from build123d import *

# Parameters (mm, degrees)
SKETCH1_W                                     = 120
SKETCH1_H                                     = 36.5
BOSS_EXTRUDE1_DEPTH                           = 3
CUT_EXTRUDE1_DEPTH                            = 4
CSK_FOR_5_OVAL_HEAD_MACHINE_SCREW1_AT_2_COUNT = 2
CSK_FOR_5_OVAL_HEAD_MACHINE_SCREW1_AT_2_PITCH = 100.75


with BuildPart() as part:
    # Sketch1 → Boss-Extrude1 (new body)
    with BuildSketch(Plane(origin=(0, 0, 0), x_dir=(1, 0, 0), z_dir=(0, 1, 0))):
        with Locations((60, -18.25)):
            Rectangle(SKETCH1_W, SKETCH1_H)
    extrude(amount=BOSS_EXTRUDE1_DEPTH)

    # Sketch2 → Cut-Extrude1 (cut, through all)
    with BuildSketch(Plane(origin=(0, 3, 0), x_dir=(1, 0, 0), z_dir=(0, 1, 0))):
        Polygon((19.25, -32.25), (100.75, -32.25), (100.75, -4.25), (60, -4.25), (19.25, -4.25), align=None)
    extrude(amount=-CUT_EXTRUDE1_DEPTH, mode=Mode.SUBTRACT)

    # Sketch6 → CSK for #5 Oval Head Machine Screw1 (revolve, cut)
    with BuildSketch(Plane(origin=(9.625, 3, 18.25), x_dir=(0, 0, 1), z_dir=(1, 0, 0))):
        Polygon((0, 0), (0, 3), (2.5499949, 3), (2.5499949, 2.7000073), (5.2500022, 0), align=None)
    csk_for_5_oval_head_machine_screw1 = revolve(axis=Axis((9.625, 9.35, 18.25), (0, -1, 0)), mode=Mode.SUBTRACT)

    # CSK for #5 Oval Head Machine Screw1 at 2: CSK for #5 Oval Head Machine Screw1 ×2
    with Locations(*[(i * CSK_FOR_5_OVAL_HEAD_MACHINE_SCREW1_AT_2_PITCH, 0, 0) for i in range(1, CSK_FOR_5_OVAL_HEAD_MACHINE_SCREW1_AT_2_COUNT)]):
        add(csk_for_5_oval_head_machine_screw1, mode=Mode.SUBTRACT)


solid = part.part
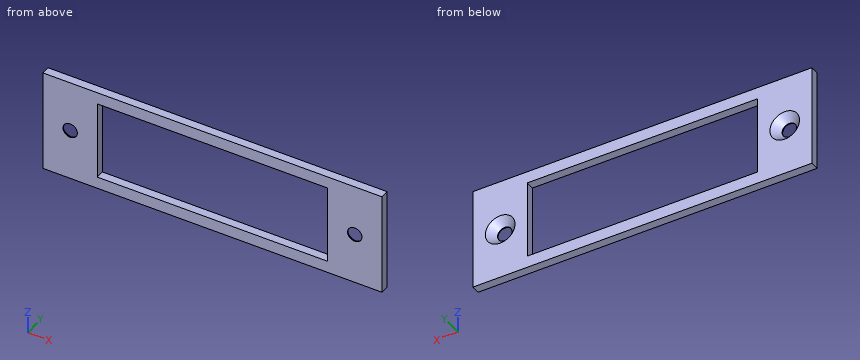
Design review of the part built by this model. Coordinates are the model's own, in mm. Round coordinates to 2 decimals unless told otherwise and drop trailing zeros. Write each loop counter-clockwise with the first axis right and the second up, starting at its lowest first coordinate (ties: lowest second). Pieces come first, ordered by that corner, then holes. Notation, with made-up numbers: (63, 78.5) - (101, 78.5) arc R25 ccw to (101, 92.5) - close; hole circle Ø1 at (-3, 29.5). An arc over 180 degrees is marked (long way). Return JSON: item names as keys, results as strings. Group by question number.
Item 1: We need section C-C on z = 18.25. Write out the cut boundary in (x, y) (3 decimals).
Item 2: Insertion check: P1, Ø8, axis at x = 18.5, z = 4, coming from the -Y side. The pin has a flat end and moves straight along its axis. Give the tip position at first contact, or say it passes through.
Item 3: For probe 1 along X at (y, z) = (0.15, 18.25) (3 decimals); probe 2 along Z at (x, y) = (95, 0.2); probe 3 along X at (y, z) = (0.2, 29), list the stretches that pass through material, from the lowest coordinate up. Write a range as [from, to].
Item 4: We need section D-D on y = 1.05. Write out the cut boundary in (x, z) (3 decimals), and give its area (3 significant figures).
Item 5: We need section B-B on z = 31. Write out the cut boundary in (x, y), and give its area (4 significant figures).
Item 6: We need section A-A on x = 60.5. Write out the cut boundary in (y, z), and give its area (3 significant figures).
Model answer:
{
 "1": {"outline": "(0, 0) - (7.075, 0) - (7.075, 0.3) - (4.375, 3) - (0, 3) - close; (12.175, 0) - (19.25, 0) - (19.25, 3) - (14.875, 3) - (12.175, 0.3) - close; (100.75, 0) - (107.825, 0) - (107.825, 0.3) - (105.125, 3) - (100.75, 3) - close; (112.925, 0) - (120, 0) - (120, 3) - (115.625, 3) - (112.925, 0.3) - close"},
 "2": {"P1": "stops at y = 0"},
 "3": {"probe 1": "x = [0, 7.075], [12.175, 19.25], [100.75, 107.825], [112.925, 120]", "probe 2": "z = [0, 4.25], [32.25, 36.5]", "probe 3": "x = [0, 19.25], [100.75, 120]"},
 "4": {"outline": "(0, 0) - (120, 0) - (120, 36.5) - (0, 36.5) - close; hole circle Ø6.6 at (9.625, 18.25); hole (19.25, 4.25) - (100.75, 4.25) - (100.75, 32.25) - (19.25, 32.25) - close; hole circle Ø6.6 at (110.375, 18.25)", "area": "2,030 mm²"},
 "5": {"outline": "(0, 0) - (19.25, 0) - (19.25, 3) - (0, 3) - close; (100.75, 0) - (120, 0) - (120, 3) - (100.75, 3) - close", "area": "115.5 mm²"},
 "6": {"outline": "(0, 0) - (3, 0) - (3, 4.25) - (0, 4.25) - close; (0, 32.25) - (3, 32.25) - (3, 36.5) - (0, 36.5) - close", "area": "25.5 mm²"}
}
